from build123d import *

# Parameters (mm, degrees)
SKETCH1_W           = 97.6
SKETCH1_H           = 66.43745389
BOSS_EXTRUDE1_DEPTH = 6
SKETCH4_W           = 24.6
SKETCH4_H           = 54
SKETCH4_H_2         = 6.218726945
SKETCH4_W_2         = 55
SKETCH4_W_3         = 18
BOSS_EXTRUDE2_DEPTH = 13.5
SKETCH5_W           = 34.693830492
SKETCH5_H           = 30
CUT_EXTRUDE1_DEPTH  = 13.5


with BuildPart() as part:
    # Sketch1 → Boss-Extrude1 (new body)
    with BuildSketch(Plane(origin=(0, 0, 0), x_dir=(1, 0, 0), z_dir=(0, 1, 0))):
        Rectangle(SKETCH1_W, SKETCH1_H)
    extrude(amount=BOSS_EXTRUDE1_DEPTH)

    # Sketch4 → Boss-Extrude2 (add)
    with BuildSketch(Plane(origin=(0, 6, 0), x_dir=(1, 0, 0), z_dir=(0, 1, 0))):
        with Locations((-36.5, 0)):
            Rectangle(SKETCH4_W, SKETCH4_H)
        with Locations((-36.5, -30.109363473)):
            Rectangle(SKETCH4_W, SKETCH4_H_2)
        with Locations((3.3, -30.109363473)):
            Rectangle(SKETCH4_W_2, SKETCH4_H_2)
        with Locations((39.8, -30.109363473)):
            Rectangle(SKETCH4_W_3, SKETCH4_H_2)
        with Locations((39.8, 0)):
            Rectangle(SKETCH4_W_3, SKETCH4_H)
        with Locations((39.8, 30.109363473)):
            Rectangle(SKETCH4_W_3, SKETCH4_H_2)
        with Locations((-36.5, 30.109363473)):
            Rectangle(SKETCH4_W, SKETCH4_H_2)
        with Locations((3.3, 30.109363473)):
            Rectangle(SKETCH4_W_2, SKETCH4_H_2)
    extrude(amount=BOSS_EXTRUDE2_DEPTH)

    # Sketch5 → Cut-Extrude1 (cut)
    with BuildSketch(Plane(origin=(0, 19.5, 0), x_dir=(1, 0, 0), z_dir=(0, 1, 0))):
        with Locations((-29.546650011, -5)):
            Rectangle(SKETCH5_W, SKETCH5_H)
    extrude(amount=-CUT_EXTRUDE1_DEPTH, mode=Mode.SUBTRACT)


solid = part.part
Work out the finished part from the listing and answer in its coordinate system (mm). A direction names the side the tool comes from. Give positions to 0.01 mm unless a question says otherwise; leave off trailing zeros. Write each loop counter-clockwise with the first axis right and the second up, starting at its lowest first coordinate (ties: lowest second). Pieces come first, ordered by that corner, then holes. Notation, with made-up numbers: M 69.5,-31.75 L 87.5,-31.75 A15 cw 87.5,-26.75 Z; hole C 81,83.25 d11. An arc over 180 degrees is marked long. Answer as CSV lines item,"result".
Q1. Given P1, Ø12, axis at x = 5, z = 9, coming from the +Y side, flat-ended and moving along its own axis, determine where the tip first touches the part or whether it passes through.
A:
P1,"stops at y = 6"
Q2. A cutting plane is placed at C-C on x = 19.5. Write down the section's boundary in (y, z), plus the area to 3 significant figures.
A:
outline,"M 0,-33.22 L 19.5,-33.22 L 19.5,-27 L 6,-27 L 6,27 L 19.5,27 L 19.5,33.22 L 0,33.22 Z"
area,"567 mm²"
Q3. The mould has two halves that part along Z. Classify faces 3 (the flat face through (-1, 10, 33.219)), 4 (the flat face through (0, 6, 0)), 5 (the flat face through (-1, 0, 0)): +Z half, -Z half, draft (parallel to the pull), parting line (faces both ways), or undercut.
A:
face 3,"+Z half"
face 4,"undercut"
face 5,"draft"
Q4. A cutting plane is placed at A-A on z = -18. Write down the section's boundary in (x, y), plus the area to 3 significant figures.
A:
outline,"M -48.8,0 L 48.8,0 L 48.8,19.5 L 30.8,19.5 L 30.8,6 L -24.2,6 L -24.2,19.5 L -48.8,19.5 Z"
area,"1,160 mm²"
Q5. Find the intervals of material crossed by probe 1 along X at (y, z) = (7.75, 0.5); probe 2 along Z at (x, y) = (-14, 12.5); probe 3 along X at (y, z) = (8.5, -25.5), in increasing order. Write a range as [from, to].
A:
probe 1,"x = [-48.8, -46.89], [30.8, 48.8]"
probe 2,"z = [-33.22, -27], [27, 33.22]"
probe 3,"x = [-48.8, -24.2], [30.8, 48.8]"
Q6. A cutting plane is placed at B-B on y = 14.5. Write down the section's boundary in (x, z), plus the area to 3 significant figures.
A:
outline,"M -48.8,-33.22 L 48.8,-33.22 L 48.8,33.22 L -48.8,33.22 Z; hole M -46.89,-10 L -24.2,-10 L -24.2,-27 L 30.8,-27 L 30.8,27 L -24.2,27 L -24.2,20 L -46.89,20 Z"
area,"2,830 mm²"
Q7. A tool of negligible diameter and unlimited length cuts with its end or side. For faces 1 (the flat face through (1, 10, -33.219)), 2 (the flat face through (-46.894, 13, 5)), from which of +Z, -Z, +X, -X, +Y, -Y can it reach the whole face along a straight path? Write none if from no direction.
A:
face 1,"-Z, +X, -X, +Y, -Y"
face 2,"+Y"
